Read the model definition and answer for the solid it produces. Units are mm, in the model's axes. Face numbers are marked on the shaded views. A direction names the side the tool comes from. Coordinates: 2 decimals unless noted, no trailing zeros. Write each loop counter-clockwise with the first axis right and the second up, starting at its lowest first coordinate (ties: lowest second). Pieces come first, ordered by that corner, then holes.
(1) Given pin 1 (1 mm diameter, centred on x = 3.5, y = 2, fed in from -Z); pin 2 (6 mm diameter, centred on x = 1.5, y = 2, fed in from -Z); pin 3 (3 mm diameter, centred on y = 3.5, z = -2, fed in from +X), each flat-ended and moving along its own axis, determine where each tip first touches the part or whether it passes through.
(2) The mould has two halves that part along X. Classify the marked faces 3, 4 and 5: +X half, -X half, draft (parallel to the pull), parting line (faces both ways), or undercut.
(3) Which of the six approach directions +Z, -Z, +X, -X, +Y, -Y give full straight-line access (tool end or side, diameter ignored) to the marked faces 1 and 2?
(4) Section A-A on y = 0 is taken. Write down the section's boundary in (x, z), then the cut area to 3 significant figures.
(5) Section D-D on z = -20 is taken. Write down the section's boundary in (x, y), then the cut area to 3 significant figures.
(6) Find the intervals of material crossed by probe 1 along Y at (x, z) = (0, -5); probe 2 along Y at (x, z) = (1, -11.25); probe 3 along X at (y, z) = (-0.25, -9.5), in increasing order.
(7) Section B-B on z = -11 is taken. Write down the section's boundary in (x, y).
from build123d import *

# Parameters (mm, degrees)
F0_R     = 5.5
F0_R_2   = 3.5
F0_R_3   = 1.5
F1_DEPTH = 2
F2_DEPTH = 27
F3_DEPTH = 12
F4_SIZE2 = 1
F4_SIZE  = 4


with BuildPart() as f1:
    # F0 (on Top) → F1 (new body)
    with BuildSketch(Plane.XY):
        Circle(F0_R)
        Circle(F0_R_2, mode=Mode.SUBTRACT)
        Circle(F0_R_2)
        Circle(F0_R_3, mode=Mode.SUBTRACT)
        Circle(F0_R_3)
    extrude(amount=F1_DEPTH)

    # F0 (on Top) → F2 (join)
    with BuildSketch(Plane.XY):
        Circle(F0_R_3)
    extrude(amount=-F2_DEPTH)

    # F0 (on Top) → F3 (join)
    with BuildSketch(Plane.XY):
        Circle(F0_R)
        Circle(F0_R_2, mode=Mode.SUBTRACT)
    extrude(amount=-F3_DEPTH)

    # F4
    f4_edges = [f1.edges().sort_by_distance(p)[0] for p in [
        (-5.5, 0, -12),
    ]]
    f4_side = f1.faces().sort_by_distance((-5.5, 0, -6))[0]
    chamfer(f4_edges, length=F4_SIZE, length2=F4_SIZE2, reference=f4_side)


solid = f1.part
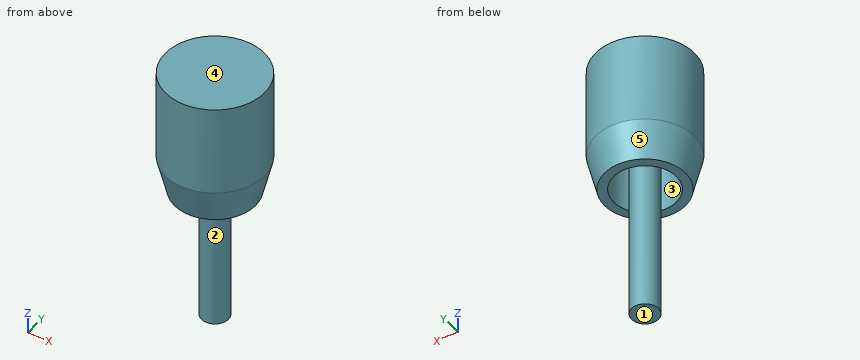
Response:
1. pin 1: stops at z = -12
1. pin 2: stops at z = -27
1. pin 3: stops at x = 5.12
2. face 3: undercut
2. face 4: draft
2. face 5: parting line
3. face 1: -Z, +X, -X, +Y, -Y
3. face 2: -Z
4. outline: (-5.5, -8) - (-4.5, -12) - (-3.5, -12) - (-3.5, 0) - (-1.5, 0) - (-1.5, -27) - (1.5, -27) - (1.5, 0) - (3.5, 0) - (3.5, -12) - (4.5, -12) - (5.5, -8) - (5.5, 2) - (-5.5, 2) - close
4. area: 147 mm2
5. outline: circle Ø3 at (0, 0)
5. area: 7.07 mm2
6. probe 1: y = -5.5 to -3.5, -1.5 to 1.5, 3.5 to 5.5
6. probe 2: y = -4.58 to -3.35, -1.12 to 1.12, 3.35 to 4.58
6. probe 3: x = -5.12 to -3.49, -1.48 to 1.48, 3.49 to 5.12
7. outline: circle Ø9.5 at (0, 0); circle Ø3 at (0, 0); hole circle Ø7 at (0, 0)
